Work out the finished part from the listing and answer in its coordinate system (mm). Coordinates: 2 decimals unless noted, no trailing zeros. Write each loop counter-clockwise with the first axis right and the second up, starting at its lowest first coordinate (ties: lowest second). Pieces come first, ordered by that corner, then holes. Notation, with made-up numbers: (-6.75, 87) - (28.25, 87) arc R31 ccw to (28.25, 116) - close; hole circle Ø9 at (47.25, 50.25). An arc over 180 degrees is marked (long way). Use one line per item in the form item = value. Start each with the question number.
Item 1: A cutting plane is placed at B-B (y = 0). Give the number of separate pieces and of enclosed holes in the cut face, then the cut area to 3 significant figures.
Item 2: Given pin 1 (4 mm diameter, centred on x = -25.82, y = -25.82, fed in from -Z); pin 2 (1 mm diameter, centred on y = 32.5, z = 3, fed in from -X), each flat-ended and moving along its own axis, determine where each tip first touches the part or whether it passes through.
Item 3: A cutting plane is placed at D-D (x = 12.7). Write down the section's boundary in (y, z).
Item 4: Consider probe 1 along X at (y, z) = (23, 1); probe 2 along Y at (x, z) = (-26, 0.75); probe 3 along X at (y, z) = (23.5, 2.75). Determine where each line is inside the solid, lowest interval first.
Item 5: Determine the mould class of faces 1 (the cylindrical face through (-11.722, 24.355, 3.219)), 2 (the flat face through (-10, 1, 6.35)), 3 (the cylindrical face through (-12.812, -24.547, 3.219)) for opening direction X: released by +X, released by -X, zero draft, split by the parting line, or undercut.
Item 6: A cutting plane is placed at A-A (x = 0). Write down the section's boundary in (y, z) (3 decimals).
Autodesk Inventor part; units mm, degrees
ref_plane "YZ Plane" through (0, 0, 0) normal (1, 0, 0) x (0, 1, 0)
ref_plane "XZ Plane" through (0, 0, 0) normal (0, 1, 0) x (-1, 0, 0)
ref_plane "XY Plane" through (0, 0, 0) normal (0, 0, 1) x (1, 0, 0)
sketch "Sketch1" plane through (0, 0, 0) normal (0, 0, 1) x (1, 0, 0)
  circle A0 centre (0, 0) radius 9.525
  circle A1 centre (0, 0) radius 31.75 construction
  circle A2 centre (-36.5125, 0) radius 4.7625 construction
  circle A3 centre (36.5125, 0) radius 4.7625 construction
  circle A4 centre (0, 0) radius 17.4625 construction
  line L0 (-36.5125, 0) -> (36.5125, 0) construction
  circle A5 centre (0, 0) radius 25.4 construction
  circle A6 centre (0, 0) radius 36.5125 construction
  line L1 (0, 36.5125) -> (0, 0) construction
  line L2 (-25.8182, 25.8182) -> (0, 0) construction
  circle A7 centre (-25.8182, 25.8182) radius 4.7625 construction
  circle A8 centre (-25.8182, -25.8182) radius 4.7625 construction
  circle A9 centre (25.8182, -25.8182) radius 4.7625 construction
  circle A10 centre (25.8182, 25.8182) radius 4.7625 construction
  circle A11 centre (0, 0) radius 41.275
  point P0 (-17.4625, 0)
  point P1 (-25.4, 0)
  point P2 (-12.7, -21.997)
  point P3 (-8.7313, -15.123)
  point P4 (12.7, -21.997)
  point P5 (8.7312, -15.123)
  point P6 (25.4, 0)
  point P7 (17.4625, 0)
  point P8 (12.7, 21.997)
  point P9 (8.7313, 15.123)
  point P10 (-12.7, 21.997)
  point P11 (-8.7312, 15.123)
  dimension "d3" = 34.925
  dimension "d18" = 50.8
  dimension "d0" = 19.05
  dimension "d1" = 63.5
  dimension "d2" = 9.525
  dimension "d21" = 360
  dimension "d30" = 45
  dimension "d33" = 360
  dimension "d37" = 360
extrude "Extrusion1" add sketch "Sketch1" along normal blind 6.35
hole "Hole2" at (-17.4625, 0, 0) at (-36.5125, 0, 0) at (36.5125, 0, 0) at (-25.4, 0, 0) at (-12.7, -21.997, 0) at (-8.7313, -15.123, 0) at (12.7, -21.997, 0) at (8.7312, -15.123, 0) at (25.4, 0, 0) at (17.4625, 0, 0) at (12.7, 21.997, 0) at (8.7313, 15.123, 0) at (-12.7, 21.997, 0) at (-8.7312, 15.123, 0) at (-25.8182, 25.8182, 0) at (25.8182, 25.8182, 0) at (25.8182, -25.8182, 0) at (-25.8182, -25.8182, 0) direction (0, 0, 1) diameter 5.1054 end through all
properties part number "GP9-003" material "Polycarbonate, Smoke"
Answer:
q1.separate_pieces = 8
q1.enclosed_holes = 0
q1.area = 209 mm²
q2.pin_1 = through
q2.pin_2 = -26.07
q3.outline = (-39.27, 0) - (-24.55, 0) - (-24.55, 6.35) - (-39.27, 6.35) - close; (-19.44, 0) - (19.44, 0) - (19.44, 6.35) - (-19.44, 6.35) - close; (24.55, 0) - (39.27, 0) - (39.27, 6.35) - (24.55, 6.35) - close
q4.probe_1 = -34.27 to -15.05, -10.35 to 10.35, 15.05 to 34.27
q4.probe_2 = -32.06 to -28.36, -23.27 to -2.48, 2.48 to 23.27, 28.36 to 32.06
q4.probe_3 = -33.93 to -26.89, -24.75 to -14.76, -10.64 to 10.64, 14.76 to 24.75, 26.89 to 33.93
q5.face_1 = undercut
q5.face_2 = zero draft
q5.face_3 = undercut
q6.outline = (-41.275, 0) - (-9.525, 0) - (-9.525, 6.35) - (-41.275, 6.35) - close; (9.525, 0) - (41.275, 0) - (41.275, 6.35) - (9.525, 6.35) - close
